Here's the drawing with two shaded views (mm, measured from the low corner). I have some questions. A direction names the side the tool comes from. Give positions to 0.01 mm unless a question says otherwise; leave off trailing zeros. Loops run counter-clockwise (first coordinate to the right, second up) from the corner with the lowest first, then second, coordinate; pieces in that order, holes last. Notation, with made-up numbers: M 48.5,47.25 L 66.5,47.25 A9 ccw 66.5,61.25 Z; hole C 31.25,60 d10. An arc over 180 degrees is marked long. Use a Markdown table: item, result. Add a question column.
1) Will this pin go through, and if not, where does the flat tip stop? pin 1 Ø6 at (x, y) = (13, 23.5) entering from +Z.
2) Suppose I cut it at B-B on x = 13. List the corners of the cut face in (y, z) for me, and give its area (3 significant figures).
3) If I drill on line 1 along Y through (x, z) = (8.5, 2.75); line 2 along X through (y, z) = (17, 6), over which ranges is the centre line in solid material (lowest first)? Write a range as [from, to].
4) Which directions (+Z, -Z, +X, -X, +Y, -Y) give clear straight access to the entire face, cutting with the end or side of a thin tool? Please do the marked faces 1 and 2.
5) Suppose I cut it at A-A on z = 2. List the corners of the cut face in (x, y) for me, and give its area (3 significant figures).
6) Suppose I cut it at D-D on y = 16. List the corners of the cut face in (x, z) for me.
7) We'd pull the mould along Y, two halves only. Please class the marked faces 3, 4 and 5: +Y half, -Y half, draft (parallel to the pull), parting line (faces both ways), or undercut.
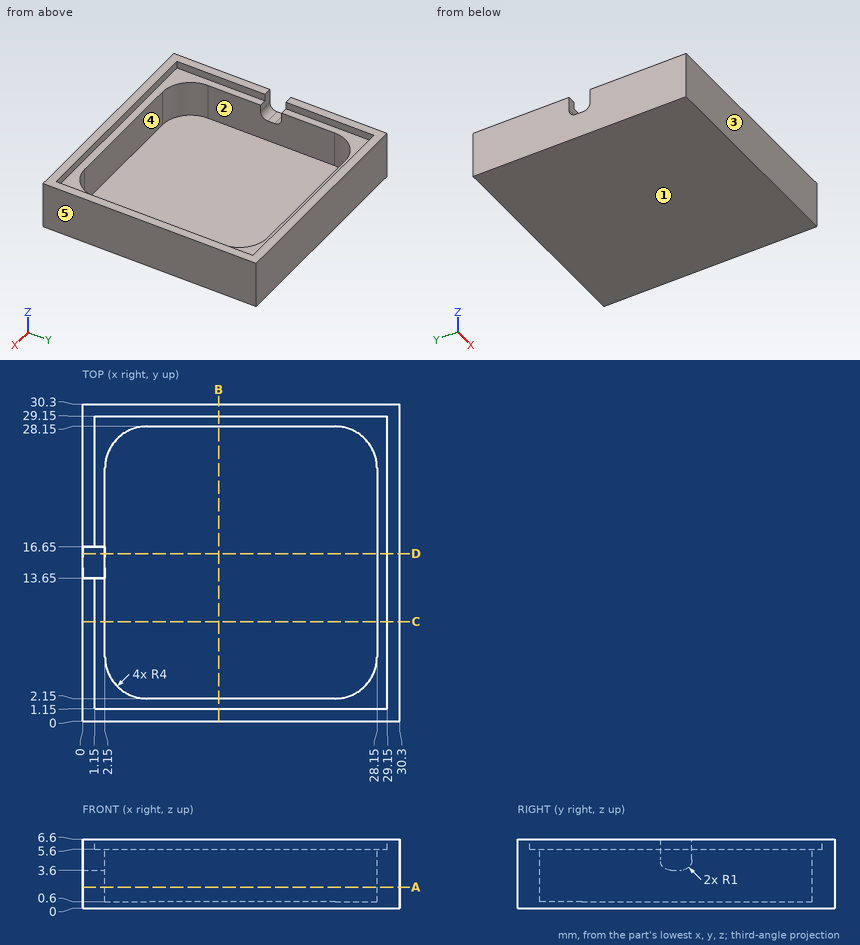
Answer block:
| question | item | result |
|---|---|---|
| 1 | pin 1 | stops at z = 0.6 |
| 2 | outline | M 0,0 L 30.3,0 L 30.3,6.6 L 29.15,6.6 L 29.15,5.6 L 28.15,5.6 L 28.15,0.6 L 2.15,0.6 L 2.15,5.6 L 1.15,5.6 L 1.15,6.6 L 0,6.6 Z |
| 2 | area | 42.0 mm^2 |
| 3 | line 1 | y = [0, 2.15], [28.15, 30.3] |
| 3 | line 2 | x = [0, 1.15], [29.15, 30.3] |
| 4 | face 1 | -Z, +X, -X, +Y, -Y |
| 4 | face 2 | +Z |
| 5 | outline | M 0,0 L 30.3,0 L 30.3,30.3 L 0,30.3 Z; hole M 2.15,6.15 A4 ccw 6.15,2.15 L 24.15,2.15 A4 ccw 28.15,6.15 L 28.15,24.15 A4 ccw 24.15,28.15 L 6.15,28.15 A4 ccw 2.15,24.15 Z |
| 5 | area | 256 mm^2 |
| 6 | outline | M 0,0 L 30.3,0 L 30.3,6.6 L 29.15,6.6 L 29.15,5.6 L 28.15,5.6 L 28.15,0.6 L 2.15,0.6 L 2.15,3.66 L 0,3.66 Z |
| 7 | face 3 | -Y half |
| 7 | face 4 | undercut |
| 7 | face 5 | draft |
